from build123d import *

# Parameters (mm, degrees)
SKETCH1_W           = 125.73
SKETCH1_H           = 76.2
SKETCH1_W_2         = 10.16
SKETCH1_H_2         = 3.302
BOSS_EXTRUDE1_DEPTH = 3.175
FILLET1_R           = 12.7
CUT_EXTRUDE2_DEPTH  = 74.577842113


with BuildPart() as part:
    # Sketch1 → Boss-Extrude1 (new body)
    with BuildSketch(Plane.XY):
        Rectangle(SKETCH1_W, SKETCH1_H)
        with Locations((-28.4988, -30.226)):
            Rectangle(SKETCH1_W_2, SKETCH1_H_2, mode=Mode.SUBTRACT)
        with Locations((28.4988, -30.226)):
            Rectangle(SKETCH1_W_2, SKETCH1_H_2, mode=Mode.SUBTRACT)
    extrude(amount=BOSS_EXTRUDE1_DEPTH)

    # Fillet1
    fillet1_edges = [part.edges().sort_by_distance(p)[0] for p in [
        (62.865, -38.1, 1.5875),
        (-62.865, -38.1, 1.5875),
        (-62.865, 38.1, 1.5875),
        (62.865, 38.1, 1.5875),
    ]]
    fillet(fillet1_edges, radius=FILLET1_R)

    # Sketch5 → Cut-Extrude2 (cut, through all)
    with BuildSketch(Plane.XY.offset(3.175)):
        with BuildLine():
            Line((2.984111333, 21.969779064), (2.984111333, -17.372056987))
            ThreePointArc((2.984111333, -17.372056987), (0, -20.35616832), (-2.984111333, -17.372056987))
            Line((-2.984111333, -17.372056987), (-2.984111333, 21.969779064))
            ThreePointArc((-2.984111333, 21.969779064), (0, 24.953890397), (2.984111333, 21.969779064))
        make_face()
        with BuildLine():
            Line((15.684111333, 21.969779064), (15.684111333, -17.372056987))
            ThreePointArc((15.684111333, -17.372056987), (12.7, -20.35616832), (9.715888667, -17.372056987))
            Line((9.715888667, -17.372056987), (9.715888667, 21.969779064))
            ThreePointArc((9.715888667, 21.969779064), (12.7, 24.953890397), (15.684111333, 21.969779064))
        make_face()
        with BuildLine():
            Line((28.384111333, 21.969779064), (28.384111333, -17.372056987))
            ThreePointArc((28.384111333, -17.372056987), (25.4, -20.35616832), (22.415888667, -17.372056987))
            Line((22.415888667, -17.372056987), (22.415888667, 21.969779064))
            ThreePointArc((22.415888667, 21.969779064), (25.4, 24.953890397), (28.384111333, 21.969779064))
        make_face()
        with BuildLine():
            Line((41.084111333, 21.969779064), (41.084111333, -17.372056987))
            ThreePointArc((41.084111333, -17.372056987), (38.1, -20.35616832), (35.115888667, -17.372056987))
            Line((35.115888667, -17.372056987), (35.115888667, 21.969779064))
            ThreePointArc((35.115888667, 21.969779064), (38.1, 24.953890397), (41.084111333, 21.969779064))
        make_face()
        with BuildLine():
            Line((53.784111333, 21.969779064), (53.784111333, -17.372056987))
            ThreePointArc((53.784111333, -17.372056987), (50.8, -20.35616832), (47.815888667, -17.372056987))
            Line((47.815888667, -17.372056987), (47.815888667, 21.969779064))
            ThreePointArc((47.815888667, 21.969779064), (50.8, 24.953890397), (53.784111333, 21.969779064))
        make_face()
        with BuildLine():
            Line((-9.715888667, 21.969779064), (-9.715888667, -17.372056987))
            ThreePointArc((-9.715888667, -17.372056987), (-12.7, -20.35616832), (-15.684111333, -17.372056987))
            Line((-15.684111333, -17.372056987), (-15.684111333, 21.969779064))
            ThreePointArc((-15.684111333, 21.969779064), (-12.7, 24.953890397), (-9.715888667, 21.969779064))
        make_face()
        with BuildLine():
            Line((-22.415888667, 21.969779064), (-22.415888667, -17.372056987))
            ThreePointArc((-22.415888667, -17.372056987), (-25.4, -20.35616832), (-28.384111333, -17.372056987))
            Line((-28.384111333, -17.372056987), (-28.384111333, 21.969779064))
            ThreePointArc((-28.384111333, 21.969779064), (-25.4, 24.953890397), (-22.415888667, 21.969779064))
        make_face()
        with BuildLine():
            Line((-35.115888667, 21.969779064), (-35.115888667, -17.372056987))
            ThreePointArc((-35.115888667, -17.372056987), (-38.1, -20.35616832), (-41.084111333, -17.372056987))
            Line((-41.084111333, -17.372056987), (-41.084111333, 21.969779064))
            ThreePointArc((-41.084111333, 21.969779064), (-38.1, 24.953890397), (-35.115888667, 21.969779064))
        make_face()
        with BuildLine():
            Line((-47.815888667, 21.969779064), (-47.815888667, -17.372056987))
            ThreePointArc((-47.815888667, -17.372056987), (-50.8, -20.35616832), (-53.784111333, -17.372056987))
            Line((-53.784111333, -17.372056987), (-53.784111333, 21.969779064))
            ThreePointArc((-53.784111333, 21.969779064), (-50.8, 24.953890397), (-47.815888667, 21.969779064))
        make_face()
    extrude(amount=-CUT_EXTRUDE2_DEPTH, mode=Mode.SUBTRACT)


solid = part.part
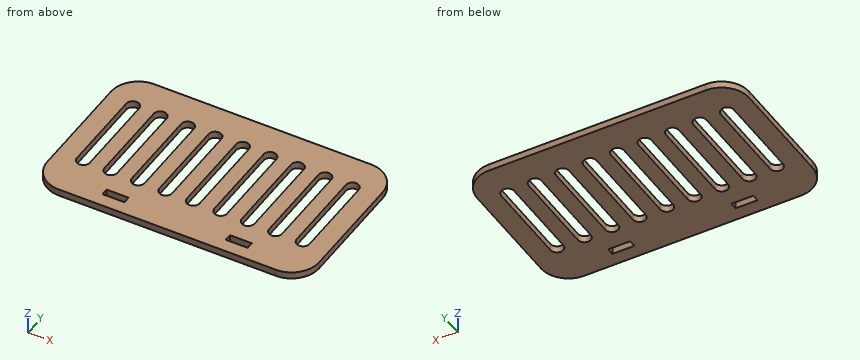
Can you work these out from the model? Positions are in its coordinate system, mm. Coordinates: 2 decimals unless noted, no trailing zeros. Loops run counter-clockwise (first coordinate to the right, second up) from the corner with the lowest first, then second, coordinate; pieces in that order, holes last. Notation, with made-up numbers: (-2, -23.75) - (52, -23.75) arc R19 ccw to (52, 12.25) - close; hole circle Ø8 at (55.5, 53.25). An arc over 180 degrees is marked (long way). Answer as a JSON object with one key per item and string values. Group by question number.
Item 1: If we section it at B-B (x = -12.7): List the corners of the cut face in (y, z) for me (3 decimals), plus the area to 3 significant figures.
Item 2: If I drill on L1, parallel to Y at x = -38, z = 1.1; L2, parallel to Y at x = 24, z = 2.95 (3 decimals); L3, parallel to Y at x = -38.5, z = 0.25, over which ranges is the centre line in solid material (lowest first)? Write a range as from..to.
Item 3: If we section it at A-A (x = 25.4): List the corners of the cut face in (y, z) for me (3 decimals).
Item 4: If we section it at C-C (y = -11.5): State how many separate pieces and enclosed holes the cut face has, plus the area to 3 significant figures.
Item 5: For pin 1 (1.6 mm diameter, centred on y = -30.5, z = 1.5, fed in from +X), with a flat end and sliding along its axis, tell me the tip position at first contact or that it passes through.
Returned:
{
 "1": {"outline": "(-38.1, 0) - (-20.356, 0) - (-20.356, 3.175) - (-38.1, 3.175) - close; (24.954, 0) - (38.1, 0) - (38.1, 3.175) - (24.954, 3.175) - close", "area": "98.1 mm²"},
 "2": {"L1": "y = -38.1..-20.35, 24.95..38.1", "L2": "y = -38.1..-31.877, -28.575..-20.007, 24.605..38.1", "L3": "y = -38.1..-20.33, 24.93..38.1"},
 "3": {"outline": "(-38.1, 0) - (-31.877, 0) - (-31.877, 3.175) - (-38.1, 3.175) - close; (-28.575, 0) - (-20.356, 0) - (-20.356, 3.175) - (-28.575, 3.175) - close; (24.954, 0) - (38.1, 0) - (38.1, 3.175) - (24.954, 3.175) - close"},
 "4": {"separate pieces": "10", "enclosed holes": "0", "area": "229 mm²"},
 "5": {"pin 1": "stops at x = 62.11"}
}
